```python
from build123d import *

# Parameters (mm, degrees)
SKETCH1_R                = 100
BOSS_EXTRUDE1_DEPTH      = 3.175
SKETCH2_R                = 17.5
CUT_EXTRUDE1_DEPTH       = 4.175
SKETCH3_R                = 3.175
CUT_EXTRUDE2_DEPTH       = 10
CUT_EXTRUDE3_DEPTH       = 3.175
FILLET1_R                = 3
CIRPATTERN1_COUNT        = 5
FILLET1_OF_CIRPATTERN1_R = 3


with BuildPart() as part:
    # Sketch1 → Boss-Extrude1 (new body)
    with BuildSketch(Plane(origin=(0, 0, 0), x_dir=(1, 0, 0), z_dir=(0, 1, 0))):
        Circle(SKETCH1_R)
    extrude(amount=BOSS_EXTRUDE1_DEPTH)

    # Sketch2 → Cut-Extrude1 (cut, through all)
    with BuildSketch(Plane(origin=(0, 3.175, 0), x_dir=(1, 0, 0), z_dir=(0, 1, 0))):
        with Locations((0, 75)):
            Circle(SKETCH2_R)
    extrude(amount=-CUT_EXTRUDE1_DEPTH, mode=Mode.SUBTRACT)

    # Sketch3 → Cut-Extrude2 (cut)
    with BuildSketch(Plane(origin=(0, 3.175, 0), x_dir=(1, 0, 0), z_dir=(0, 1, 0))):
        Circle(SKETCH3_R)
    extrude(amount=-CUT_EXTRUDE2_DEPTH, mode=Mode.SUBTRACT)

    # Sketch4 → Cut-Extrude3 (cut)
    with BuildSketch(Plane(origin=(0, 3.175, 0), x_dir=(1, 0, 0), z_dir=(0, 1, 0))):
        with BuildLine():
            Line((3.817355, 49.854065), (3.817355, 12.059345))
            Line((3.817355, 12.059345), (10.289491, 7.357063))
            Line((10.289491, 7.357063), (46.234406, 19.036274))
            ThreePointArc((46.234406, 19.036274), (29.389263, 40.45085), (3.817355, 49.854065))
        make_face()
    cut_extrude3 = extrude(amount=-CUT_EXTRUDE3_DEPTH, mode=Mode.SUBTRACT)

    # Fillet1
    fillet1_edges = [part.edges().sort_by_distance(p)[0] for p in [
        (3.817355, 1.5875, -49.854065),
        (46.234406, 1.5875, -19.036274),
        (10.289491, 1.5875, -7.357063),
        (3.817355, 1.5875, -12.059345),
    ]]
    fillet(fillet1_edges, radius=FILLET1_R)

    # CirPattern1: Cut-Extrude3 ×5 about axis
    cirpattern1_axis = Axis((0, 0, 0), (0, 1, 0))
    for i in range(1, CIRPATTERN1_COUNT):
        add(cut_extrude3.rotate(cirpattern1_axis, i * 360 / CIRPATTERN1_COUNT), mode=Mode.SUBTRACT)

    # Fillet1 of CirPattern1
    fillet1_of_cirpattern1_edges = [part.edges().sort_by_distance(p)[0] for p in [
        (-46.234406, 1.5875, -19.036274),
        (-3.817355, 1.5875, -49.854065),
        (-3.817355, 1.5875, -12.059345),
        (-10.289491, 1.5875, -7.357063),
        (-32.391789, 1.5875, 38.089001),
        (-48.593661, 1.5875, -11.775233),
        (-12.648746, 1.5875, -0.096022),
        (-10.17661, 1.5875, 7.51243),
        (26.215179, 1.5875, 42.576571),
        (-26.215179, 1.5875, 42.576571),
        (-4, 1.5875, 12),
        (4, 1.5875, 12),
        (48.593661, 1.5875, -11.775233),
        (32.391789, 1.5875, 38.089001),
        (10.17661, 1.5875, 7.51243),
        (12.648746, 1.5875, -0.096022),
    ]]
    fillet(fillet1_of_cirpattern1_edges, radius=FILLET1_OF_CIRPATTERN1_R)


solid = part.part
```
The listing builds one solid part. Answer for the finished solid, in the listing's coordinates (mm). A direction names the side the tool comes from. Coordinates: 2 decimals unless noted, no trailing zeros. Write each loop counter-clockwise with the first axis right and the second up, starting at its lowest first coordinate (ties: lowest second). Pieces come first, ordered by that corner, then holes. Notation, with made-up numbers: (35, 44.5) - (58, 44.5) arc R24 cw to (58, 63.5) - close; hole circle Ø7 at (85.25, 29). An arc over 180 degrees is marked (long way). Return JSON: item names as keys, results as strings. Group by question number.
Q1. The part is cut by section D-D on x = 73.5. Write down the section's boundary in (y, z) (3 decimals), and give its area (3 significant figures).
Q2. Which of the six approach directions +Z, -Z, +X, -X, +Y, -Y give full straight-line access (tool end or side, diameter ignored) to faces 1 (the cylindrical face through (-47.656, 1.61, 15.129)), 2 (the flat face through (-1, 0, -24))?
Q3. The part is cut by section C-C on y = 1.8. State how many separate pieces and enclosed holes the cut face has, and give its area (3 significant figures).
Q4. Find the intervals of material crossed by line 1 along Z through (x, y) = (0, 2.35) (3 decimals); line 2 along X through (y, z) = (1.15, 28.5); line 3 along X through (y, z) = (1.1, 0) (3 decimals), in increasing order. Write a range as [from, to].
Q5. The part is cut by section A-A on x = 0. Write down the section's boundary in (y, z) (3 decimals), and give its area (3 significant figures).
Q6. A flat-ended cylindrical pin translates along its axis: pin 1 Ø1.6 at (y, z) = (1, -30.5) entering from -X. Find the tip coordinate at first contact, or state that the pin passes through.
Q7. The part is cut by section B-B on z = -75. Write down the section's boundary in (x, y) (3 decimals), and give its area (3 significant figures).
Q8. For a pull along Z with two mould halves and no side action, classify faces 3 (the flat face through (-1, 3.175, -24)), 4 (the flat face through (14.71, 1.61, 26.74)), 5 (the cylindrical face through (95.38, 1.57, -30.04)), 6 (the flat face through (-27.614, 1.61, -12.986)) as +Z half, -Z half, draft (parallel to the pull), parting line (faces both ways), or undercut.
Evaluation:
{
 "1": {"outline": "(0, -67.807) - (3.175, -67.807) - (3.175, 67.807) - (0, 67.807) - close", "area": "431 mm2"},
 "2": {"face 1": "+Y, -Y", "face 2": "+Z, -Z, +X, -X, -Y"},
 "3": {"separate pieces": "1", "enclosed holes": "7", "area": "24,500 mm2"},
 "4": {"line 1": "z = [-100, -92.5], [-57.5, -3.175], [3.175, 12], [50, 100]", "line 2": "x = [-95.85, -41.08], [-25.42, -15.99], [15.99, 25.42], [41.08, 95.85]", "line 3": "x = [-100, -50], [-13.085, -3.175], [3.175, 13.085], [50, 100]"},
 "5": {"outline": "(0, -100) - (3.175, -100) - (3.175, -92.5) - (0, -92.5) - close; (0, -57.5) - (3.175, -57.5) - (3.175, -3.175) - (0, -3.175) - close; (0, 3.175) - (3.175, 3.175) - (3.175, 12) - (0, 12) - close; (0, 50) - (3.175, 50) - (3.175, 100) - (0, 100) - close", "area": "383 mm2"},
 "6": {"pin 1": "stops at x = -95.49"},
 "7": {"outline": "(-66.144, 0) - (-17.5, 0) - (-17.5, 3.175) - (-66.144, 3.175) - close; (17.5, 0) - (66.144, 0) - (66.144, 3.175) - (17.5, 3.175) - close", "area": "309 mm2"},
 "8": {"face 3": "draft", "face 4": "undercut", "face 5": "parting line", "face 6": "undercut"}
}
